Work out the finished part from the listing and answer in its coordinate system (mm). Face numbers are marked on the shaded views. A direction names the side the tool comes from. Coordinates: 2 decimals unless noted, no trailing zeros. Write each loop counter-clockwise with the first axis right and the second up, starting at its lowest first coordinate (ties: lowest second). Pieces come first, ordered by that corner, then holes. Notation, with made-up numbers: (26.25, 24.5) - (40.25, 24.5) arc R26 cw to (40.25, 38.5) - close; hole circle Ø1 at (-30, -38.5). An arc over 180 degrees is marked (long way). Use one line per item in the form item = value. Start each with the question number.
Item 1: A cutting plane is placed at C-C (x = 40). Write down the section's boundary in (y, z), then the cut area to 3 significant figures.
Item 2: Given pin 1 (10 mm diameter, centred on x = 45.5, z = -15.5, fed in from +Y); pin 2 (10 mm diameter, centred on x = 38, y = 14, fed in from -Z); pin 3 (12.5 mm diameter, centred on x = 9.5, y = 66.5, fed in from -Z), each flat-ended and moving along its own axis, determine where each tip first touches the part or whether it passes through.
Item 3: Determine the mould class of the marked faces 3, 4 and 5 for opening direction Z: released by +Z, released by -Z, zero draft, split by the parting line, or undercut.
Item 4: For the marked faces 1 and 2, determine the directions among +Z, -Z, +X, -X, +Y, -Y from which every point of the face is accessible in a straight line to the end or side of a thin tool.
Item 5: A cutting plane is placed at A-A (y = 0). Write down the section's boundary in (x, z).
Item 6: A cutting plane is placed at B-B (z = 0). Write down the section's boundary in (x, y).
Item 7: Consider probe 1 along Z at (x, y) = (-25, 0); probe 2 along Y at (x, z) = (-6, -3.5); probe 3 along Y at (x, z) = (22, -20). Determine where each line is inside the solid, lowest interval first.
from build123d import *

# Parameters (mm, degrees)
F0_R     = 25.4
F1_DEPTH = 61.35


with BuildPart() as f1:
    # F0 (on Right) → F1 (new body, symmetric)
    with BuildSketch(Plane.YZ):
        Polygon((75, 38.1), (-75, 38.1), (-75, 31.75), (-50, 31.75), (-1.82e-08, 31.75), (50, 31.75), (75, 31.75), align=None)
        with BuildLine():
            Line((-1.82e-08, 31.75), (-50, 31.75))
            Line((-50, 31.75), (-28.7355912274, -13.5028995706))
            ThreePointArc((-28.7355912274, -13.5028995706), (-26.8027942749, 17.0197743538), (-1.82e-08, 31.75))
        make_face()
        with BuildLine():
            ThreePointArc((31.75, 0), (22.4506402963, 22.4506403091), (-1.82e-08, 31.75))
            ThreePointArc((-1.82e-08, 31.75), (-26.8027942749, 17.0197743538), (-28.7355912274, -13.5028995706))
            ThreePointArc((-28.7355912274, -13.5028995706), (0, -31.75), (28.7355912274, -13.5028995706))
            ThreePointArc((28.7355912274, -13.5028995706), (30.9872354484, -6.9176397178), (31.75, 0))
        make_face()
        Circle(F0_R, mode=Mode.SUBTRACT)
        with BuildLine():
            Line((28.7355912274, -13.5028995706), (50, 31.75))
            Line((50, 31.75), (-1.82e-08, 31.75))
            ThreePointArc((-1.82e-08, 31.75), (22.4506402963, 22.4506403091), (31.75, 0))
            ThreePointArc((31.75, 0), (30.9872354484, -6.9176397178), (28.7355912274, -13.5028995706))
        make_face()
    extrude(amount=F1_DEPTH, both=True)


solid = f1.part
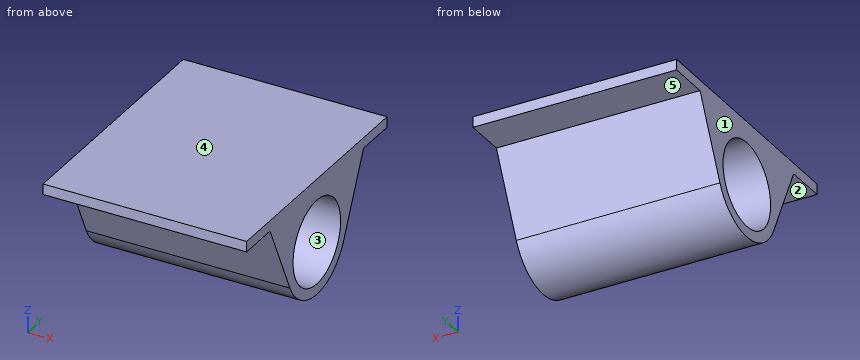
Answer:
q1.outline = (-75, 31.75) - (-50, 31.75) - (-28.74, -13.5) arc R31.75 ccw to (28.74, -13.5) - (50, 31.75) - (75, 31.75) - (75, 38.1) - (-75, 38.1) - close; hole circle Ø50.8 at (0, 0)
q1.area = 3,240 mm²
q2.pin_1 = 30.15
q2.pin_2 = -30.45
q2.pin_3 = 31.75
q3.face_3 = undercut
q3.face_4 = released by +Z
q3.face_5 = released by -Z
q4.face_1 = +Z, -Z, -X, +Y, -Y
q4.face_2 = -Z, +X, -X, -Y
q5.outline = (-61.35, -31.75) - (61.35, -31.75) - (61.35, -25.4) - (-61.35, -25.4) - close; (-61.35, 25.4) - (61.35, 25.4) - (61.35, 38.1) - (-61.35, 38.1) - close
q6.outline = (-61.35, -35.08) - (61.35, -35.08) - (61.35, -25.4) - (-61.35, -25.4) - close; (-61.35, 25.4) - (61.35, 25.4) - (61.35, 35.08) - (-61.35, 35.08) - close
q7.probe_1 = -31.75 to -25.4, 25.4 to 38.1
q7.probe_2 = -33.44 to -25.16, 25.16 to 33.44
q7.probe_3 = -24.66 to -15.66, 15.66 to 24.66
